Autodesk Inventor part; units mm, degrees
ref_plane "YZ Plane" through (0, 0, 0) normal (1, 0, 0) x (0, 1, 0)
ref_plane "XZ Plane" through (0, 0, 0) normal (0, 1, 0) x (-1, 0, 0)
ref_plane "XY Plane" through (0, 0, 0) normal (0, 0, 1) x (1, 0, 0)
sketch "Sketch1" plane through (0, 0, 0) normal (0, 1, 0) x (-1, 0, 0)
  circle A0 centre (0, 0) radius 10
  dimension "d0" = 20
extrude "Extrusion1" add sketch "Sketch1" along normal blind 50
sketch "Sketch2" plane through (0, 50, 0) normal (0, 1, 0) x (1, 0, 0)
  circle A0 centre (0, 0) radius 17.5
  dimension "d3" = 35
extrude "Extrusion2" add sketch "Sketch2" along normal blind 13
sketch "Sketch3" plane through (0, 63, 0) normal (0, 1, 0) x (1, 0, 0)
  circle A0 centre (0, 0) radius 17
  dimension "d6" = 34
extrude "Extrusion3" add sketch "Sketch3" along normal blind 15
sketch "Sketch4" plane through (0, 78, 0) normal (0, 1, 0) x (1, 0, 0)
  circle A0 centre (0, 0) radius 20
  dimension "d9" = 40
extrude "Extrusion4" add sketch "Sketch4" along normal blind 4
sketch "Sketch5" plane through (0, 82, 0) normal (0, 1, 0) x (1, 0, 0)
  point P0 (0, 0)
properties part number "estop"
Source: CAD feature listing. Evaluate the final solid. Frame: model axes, mm. A direction names the side the tool comes from. Coordinates: 2 decimals unless noted, no trailing zeros. Order: outer loops, then holes, each group sorted by start corner. A loop starts at its lowest first (then second) coordinate and runs counter-clockwise, first axis right, second up. Notation, with made-up numbers: M 84.5,37 L 99.5,37 A11 ccw 99.5,46 Z; hole C 51,64.25 d1. An arc over 180 degrees is marked long. Write each question's results on one line, items separated by ' | '. Start each with the question number.
1) Draft query along Y for faces 4 (the face through (0, 82, 0)), 5 (the face through (0, 0, 0)), 6 (the face through (-3, 63, -17)). Return one class per face: released by +Y, released by -Y, zero draft, split by the parting line, or undercut.
2) Section query A-A (z = 0). Return the cut outline in (x, y).
3) Contact query for flat-ended pins moving along their axis: pin 1 Ø3 at (y, z) = (66, 3.5) entering from +X; pin 2 Ø8 at (x, y) = (15.5, 73) entering from -Z; pin 3 Ø4 at (y, z) = (12.5, -0.5) entering from +X. Output: stop coordinate, or through.
4) Section query C-C (y = 62). Return the cut outline in (x, z), plus the area to 3 significant figures.
5) Access query for faces 1 (the face through (2.17, 24.65, 9.76)), 2 (the face through (9.139, 70.395, 14.334)), 3 (the face through (-4.336, 79.972, -19.524)). Directions: +Z, -Z, +X, -X, +Y, -Y. A direction counts if a zero-diameter tool reaches every point of the face in a straight line with its end or side. Return the directions, or none.
6) Section query B-B (x = 0). Return the cut outline in (y, z).
7) Section query D-D (x = 11.5). Return the cut outline in (y, z), plus the area to 3 significant figures.
8) Line query: line 1 (Y direction, x = -7, z = 13); line 2 (Z direction, x = 0, y = 46); line 3 (Z direction, x = -0.5, y = 52). Output: solid intervals per line, ascending. Write a range as from..to.
Answers:
1) face 4: released by +Y | face 5: released by -Y | face 6: undercut
2) outline: M -20,78 L -17,78 L -17,63 L -17.5,63 L -17.5,50 L -10,50 L -10,0 L 10,0 L 10,50 L 17.5,50 L 17.5,63 L 17,63 L 17,78 L 20,78 L 20,82 L -20,82 Z
3) pin 1: stops at x = 16.88 | pin 2: stops at z = -12.52 | pin 3: stops at x = 10
4) outline: C 0,0 d35 | area: 962 mm^2
5) face 1: -Y | face 2: none | face 3: +Y, -Y
6) outline: M 0,-10 L 50,-10 L 50,-17.5 L 63,-17.5 L 63,-17 L 78,-17 L 78,-20 L 82,-20 L 82,20 L 78,20 L 78,17 L 63,17 L 63,17.5 L 50,17.5 L 50,10 L 0,10 Z
7) outline: M 50,-13.19 L 63,-13.19 L 63,-12.52 L 78,-12.52 L 78,-16.36 L 82,-16.36 L 82,16.36 L 78,16.36 L 78,12.52 L 63,12.52 L 63,13.19 L 50,13.19 Z | area: 849 mm^2
8) line 1: y = 50..82 | line 2: z = -10..10 | line 3: z = -17.49..17.49
